Could you check a few things on this model? Use its own coordinates, in mm. A direction names the side the tool comes from. Round coordinates to 2 decimals unless told otherwise and drop trailing zeros. Write each loop counter-clockwise with the first axis right and the second up, starting at its lowest first coordinate (ties: lowest second). Pieces come first, ordered by that corner, then holes. Notation, with made-up numbers: M -7.75,70 L 48.25,70 A19 ccw 48.25,91 Z; hole C 3.5,33.5 d2. An arc over 180 degrees is marked long. One line per question, with ' | ' between items. Start each with the question number.
```python
from build123d import *

# Parameters (mm, degrees)
CROQUIS1_R              = 1.625
SALIENTE_EXTRUIR1_DEPTH = 2.5
SALIENTE_EXTRUIR2_DEPTH = 1.58
SALIENTE_EXTRUIR3_START = 3.5
CROQUIS3_R              = 1.625
SALIENTE_EXTRUIR3_DEPTH = 3.5
SALIENTE_EXTRUIR4_START = 1.5
CROQUIS5_R              = 1.625
SALIENTE_EXTRUIR4_DEPTH = 1.5
CORTAR_EXTRUIR1_REACH   = 129.692
CROQUIS6_W              = 3.24530053
CROQUIS6_H              = 1.58
SALIENTE_EXTRUIR5_START = -2.5
CROQUIS7_W              = 1.25469947
CROQUIS7_H              = 9.25469947
SALIENTE_EXTRUIR5_DEPTH = 2.5
CROQUIS8_R              = 3.35997123
CORTAR_EXTRUIR2_DEPTH   = 1.8
CORTAR_EXTRUIR2_DRAFT   = -44
CORTAR_EXTRUIR3_DEPTH   = 2.5


with BuildPart() as part:
    # Croquis1 → Saliente-Extruir1 (new body)
    with BuildSketch(Plane.XY):
        Polygon((-126.24514053, -73.999935), (-113.25453947, -73.999935), (-113.25453947, -64.74523553), (-121.99984, -55.999935), (-126.24514053, -55.999935), (-126.24514053, -57.499935), (-122.49514053, -57.499935), (-122.49514053, -64.74523553), (-126.24514053, -64.74523553), align=None)
        with Locations((-123.49984, -70.499935)):
            Circle(CROQUIS1_R, mode=Mode.SUBTRACT)
    extrude(amount=SALIENTE_EXTRUIR1_DEPTH)

    # Croquis2 → Saliente-Extruir2 (add)
    with BuildSketch(Plane(origin=(0, 0, 0), x_dir=(-1, 0, 0), z_dir=(0, 0, -1))):
        Polygon((119.99984, -57.999935), (119.99984, -71.999935), (121.99984, -73.999935), (113.25453947, -73.999935), (113.25453947, -64.74523553), align=None)
    extrude(amount=SALIENTE_EXTRUIR2_DEPTH)

    # Croquis3 → Saliente-Extruir3 (add)
    # profile 1 of 2: a face of its own
    with BuildSketch(Plane(origin=(0, 0, -1.58), x_dir=(-1, 0, 0), z_dir=(0, 0, -1)).offset(SALIENTE_EXTRUIR3_START)):
        Polygon((113.25453947, -73.999935), (113.25453947, -64.74523553), (115.25453947, -62.74523553), (115.25453947, -73.999935), align=None)
    # profile 2 of 2: a face of its own
    with BuildSketch(Plane(origin=(0, 0, -1.58), x_dir=(-1, 0, 0), z_dir=(0, 0, -1)).offset(SALIENTE_EXTRUIR3_START)):
        Polygon((119.25453947, -73.999935), (121.99984, -73.999935), (126.24514053, -73.999935), (126.24514053, -64.74523553), (126.24514053, -55.999935), (121.99984, -55.999935), (119.99984, -57.999935), (119.25453947, -58.74523553), align=None)
        with Locations(Location((123.49984, -70.499935, 0), (0, 0, 180))):
            Circle(CROQUIS3_R, mode=Mode.SUBTRACT)
    extrude(amount=-SALIENTE_EXTRUIR3_DEPTH)

    # Croquis5 → Saliente-Extruir4 (add)
    with BuildSketch(Plane(origin=(0, 0, -5.08), x_dir=(-1, 0, 0), z_dir=(0, 0, -1)).offset(SALIENTE_EXTRUIR4_START)):
        Polygon((113.25453947, -73.999935), (126.24514053, -73.999935), (126.24514053, -55.999935), (121.99984, -55.999935), (113.25453947, -64.74523553), align=None)
        with Locations(Location((123.49984, -70.499935, 0), (0, 0, 180))):
            Circle(CROQUIS5_R, mode=Mode.SUBTRACT)
    extrude(amount=-SALIENTE_EXTRUIR4_DEPTH)

    # Cortar-Extruir1: up to this plane
    cortar_extruir1_end = Plane(origin=(-113.25453947, -64.74523553, 2.5), z_dir=(-0.7071067811865476, -0.7071067811865476, 0))
    # Croquis6 → Cortar-Extruir1 (cut, up to the surface)
    with BuildSketch(Plane.XZ.offset(73.999935), mode=Mode.PRIVATE) as cortar_extruir1_sk1:
        with Locations((-120.377189735, -0.79)):
            Rectangle(CROQUIS6_W, CROQUIS6_H)
    cortar_extruir1_tool1 = split(extrude(cortar_extruir1_sk1.sketch, amount=-CORTAR_EXTRUIR1_REACH, mode=Mode.PRIVATE), bisect_by=cortar_extruir1_end, keep=Keep.BOTH, mode=Mode.PRIVATE)
    add(cortar_extruir1_tool1.solids().sort_by_distance((-120.37719, -73.999935, -0.79))[0], mode=Mode.SUBTRACT)

    # Croquis7 → Saliente-Extruir5 (add)
    with BuildSketch(Plane.XY.offset(2.5).offset(SALIENTE_EXTRUIR5_START)):
        with Locations((-126.872490265, -69.372585265)):
            Rectangle(CROQUIS7_W, CROQUIS7_H)
    extrude(amount=SALIENTE_EXTRUIR5_DEPTH)


with BuildPart() as cortar_extruir2_tool:
    # Croquis8 → Cortar-Extruir2 (with draft: the straight prism first)
    with BuildSketch(Plane.XY.offset(2.5)):
        with Locations((-123.49984, -70.499935)):
            Circle(CROQUIS8_R)
    extrude(amount=-CORTAR_EXTRUIR2_DEPTH)
    # Cortar-Extruir2: the draft: its side faces are tilted about the plane it starts from
    cortar_extruir2_sides = [cortar_extruir2_tool.faces().sort_by_distance(p)[0] for p in [
        (-126.85981123, -70.499935, 1.6),
    ]]
    draft(cortar_extruir2_sides, Plane.XY.offset(2.5), CORTAR_EXTRUIR2_DRAFT)


with BuildPart() as part_1:
    add(part.part)

    # Cortar-Extruir2: cut by cortar_extruir2_tool
    add(cortar_extruir2_tool.part, mode=Mode.SUBTRACT)

    # Croquis9 → Cortar-Extruir3 (cut)
    with BuildSketch(Plane(origin=(0, 0, -6.58), x_dir=(-1, 0, 0), z_dir=(0, 0, -1))):
        Polygon((120.75453947, -72.084935), (123.49984, -73.669935), (124.071416766, -73.999935), (126.24514053, -73.999935), (126.24514053, -72.084935), (126.24514053, -68.914935), (123.49984, -67.329935), (120.75453947, -68.914935), align=None)
    extrude(amount=-CORTAR_EXTRUIR3_DEPTH, mode=Mode.SUBTRACT)


solid = part_1.part
```
1. Suppose I cut it at C-C (x = -118.5). Write out the boundary of the cut face in (y, z), and give its area (3 significant figures).
2. If we mould it in two halves opening along X, with no side actions, what happens to faces 1 (the face through (-123, -67, 0)), 2 (the face through (-117, -68, -1.58)), 3 (the face through (-127.5, -69, 1))? For each: released by +X, released by -X, zero draft, split by the parting line, or undercut.
3. I'm going to push flat-ended pins straight in: P1, Ø4, axis at y = -66.5, z = -3.5, coming from the -X side; P2, Ø4, axis at x = -123.5, y = -70.5, coming from the +Z side; P3, Ø0.8, axis at y = -63, z = 1.5, coming from the -X side. Where does each tip first touch, or does it pass through?
4. I need wall thicknesses on line 1 along Z through (x, y) = (-116.25, -62.5); line 2 along X through (y, z) = (-68.5, -3); line 3 along X through (y, z) = (-71.75, -3.5). Which ranges of each line are inside material? Lowest first, please. Write a range as from..to.
5. Suppose I cut it at D-D (y = -58.5). Write out the boundary of the cut face in (x, z).
6. Which directions (+Z, -Z, +X, -X, +Y, -Y) give clear straight access to the entire face, cutting with the end or side of a thin tool? Please do faces 4 (the face through (-115.255, -68, -3)), 5 (the face through (-125, -72, -4.08)), 6 (the face through (-126.245, -63, -4)), 7 (the face through (-122.495, -61, 1)).
7. Suppose I cut it at B-B (z = -2.25). Write out the boundary of the cut face in (x, y) (3 decimals).
8. Suppose I cut it at A-A (y = -65.5). Write out the boundary of the cut face in (x, z), and give its area (3 significant figures).
Computed:
1) outline: M -74,-6.58 L -59.5,-6.58 L -59.5,-5.08 L -74,-5.08 Z; M -74,-1.58 L -59.5,-1.58 L -59.5,2.5 L -74,2.5 Z | area: 80.9 mm²
2) face 1: zero draft | face 2: undercut | face 3: released by -X
3) P1: stops at x = -126.25 | P2: stops at z = 1.09 | P3: stops at x = -122.5
4) line 1: z = -6.58..-5.08, -1.58..2.5 | line 2: x = -126.25..-119.25, -115.25..-113.25 | line 3: x = -126.25..-124.54, -122.46..-119.25, -115.25..-113.25
5) outline: M -126.25,-6.58 L -119.5,-6.58 L -119.5,-1.58 L -126.25,-1.58 Z; M -122.5,0 L -119.5,0 L -119.5,2.5 L -122.5,2.5 Z
6) face 4: +Y, -Y | face 5: -Z | face 6: -Z, -X, +Y, -Y | face 7: +Z, -X
7) outline: M -126.245,-74 L -119.255,-74 L -119.255,-58.745 L -122,-56 L -126.245,-56 Z; M -115.255,-74 L -113.255,-74 L -113.255,-64.745 L -115.255,-62.745 Z; hole C -123.5,-70.5 d3.25
8) outline: M -127.5,0 L -118.75,0 L -118.75,-1.58 L -115.25,-1.58 L -115.25,-5.08 L -119.25,-5.08 L -119.25,-1.58 L -126.25,-1.58 L -126.25,-6.58 L -113.25,-6.58 L -113.25,2.5 L -127.5,2.5 Z | area: 95.3 mm²
